Model file for the job. Use its own axes, mm. A direction names the side the tool comes from. Give positions to 0.01 mm unless a question says otherwise; leave off trailing zeros. Order: outer loops, then holes, each group sorted by start corner. A loop starts at its lowest first (then second) coordinate and runs counter-clockwise, first axis right, second up. Notation, with made-up numbers: M 49,2 L 82,2 A27 ccw 82,37 Z; hole C 1,58 d3. An arc over 180 degrees is marked long. Return JSON: item names as keys, results as strings. Group by question number.
1. Two-plate mould, pull along X, no slides. Class faces 1 (the face through (85, -104, 48.006)), 2 (the face through (-113.792, -2, 24)), 3 (the face through (11.101, -108, 43)): released by +X, released by -X, zero draft, split by the parting line, or undercut.
2. Pin check, flat tips, straight feed: pin 1 (6.5 mm diameter, centred on x = -2.5, y = 106.5, fed in from +Z); pin 2 (1.5 mm diameter, centred on x = 43.5, y = -5.5, fed in from +Z); pin 3 (1 mm diameter, centred on x = -71, y = -76.5, fed in from -Z). Stop position of each tip, or through.
3. 3-axis set-ups, long thin cutter, end or side, ignore diameter. For faces 4 (the face through (113.792, -2, 24)), 5 (the face through (107, 13.716, 43)), 6 (the face through (0, -101.092, 35)), 7 (the face through (-3, 108, 38.481)): which of +Z, -Z, +X, -X, +Y, -Y reach the whole face in a straight line?
4. Slice it at B-B on y = 61. List the corners of the cut face in (x, z), then the cut area to 3 significant figures.
5. Slice it at A-A on z = 27. List the corners of the cut face in (x, y) (1 decimal).
6. Wall check: probe 1 along Y at (x, z) = (70, 44); probe 2 along Z at (x, y) = (-9, 66.5). Give the ranges that are in metal, low to high. Write a range as [from, to].
from build123d import *

# Parameters (mm, degrees)
F0_W     = 227.584
F0_H     = 227.584
F1_DEPTH = 48.006
F3_DEPTH = 25.908
F4_W     = 12.7
F4_H     = 27.432
F4_W_2   = 27.432
F4_H_2   = 12.7
F4_H_3   = 13.716
F5_DEPTH = 9.525


with BuildPart() as f1:
    # F0 (on Top) → F1 (new body)
    with BuildSketch(Plane.XY):
        Rectangle(F0_W, F0_H)
    extrude(amount=F1_DEPTH)

    # F2 (on face) → F3 (cut)
    with BuildSketch(Plane.XY.offset(48.006)):
        with BuildLine():
            Line((86.8045, 101.092), (-88.392, 101.092))
            ThreePointArc((-88.392, 101.092), (-97.372256, 97.372256), (-101.092, 88.392))
            Line((-101.092, 88.392), (-101.092, -86.8045))
            ThreePointArc((-101.092, -86.8045), (-96.907288, -96.907288), (-86.8045, -101.092))
            Line((-86.8045, -101.092), (88.392, -101.092))
            ThreePointArc((88.392, -101.092), (97.372256, -97.372256), (101.092, -88.392))
            Line((101.092, -88.392), (101.092, 86.8045))
            ThreePointArc((101.092, 86.8045), (96.907288, 96.907288), (86.8045, 101.092))
        make_face()
    extrude(amount=-F3_DEPTH, mode=Mode.SUBTRACT)

    # F4 (on face) → F5 (cut)
    with BuildSketch(Plane.XY.offset(48.006)):
        with Locations((-107.442, 0)):
            Rectangle(F4_W, F4_H)
        with Locations((-2.614738, 107.442)):
            Rectangle(F4_W_2, F4_H_2)
        with Locations((107.442, 6.858)):
            Rectangle(F4_W, F4_H_3)
        with Locations((107.442, -6.858)):
            Rectangle(F4_W, F4_H_3)
        with Locations((-2.614738, -107.442)):
            Rectangle(F4_W_2, F4_H_2)
    extrude(amount=-F5_DEPTH, mode=Mode.SUBTRACT)


solid = f1.part
Result:
{
 "1": {"face 1": "zero draft", "face 2": "released by -X", "face 3": "undercut"},
 "2": {"pin 1": "stops at z = 38.48", "pin 2": "stops at z = 22.1", "pin 3": "stops at z = 0"},
 "3": {"face 4": "+Z, -Z, +X, +Y, -Y", "face 5": "+Z, +X, -X", "face 6": "+Z", "face 7": "+Z, +Y, -Y"},
 "4": {"outline": "M -113.79,0 L 113.79,0 L 113.79,48.01 L 101.09,48.01 L 101.09,22.1 L -101.09,22.1 L -101.09,48.01 L -113.79,48.01 Z", "area": "5,690 mm2"},
 "5": {"outline": "M -113.8,-113.8 L 113.8,-113.8 L 113.8,113.8 L -113.8,113.8 Z; hole M -101.1,-86.8 A14.3 ccw -86.8,-101.1 L 88.4,-101.1 A12.7 ccw 101.1,-88.4 L 101.1,86.8 A14.3 ccw 86.8,101.1 L -88.4,101.1 A12.7 ccw -101.1,88.4 Z"},
 "6": {"probe 1": "y = [-113.79, -101.09], [101.09, 113.79]", "probe 2": "z = [0, 22.1]"}
}
